Verification items for the finished model (mm, model axes). A direction names the side the tool comes from. Coordinates: 2 decimals unless noted, no trailing zeros. Loops run counter-clockwise (first coordinate to the right, second up) from the corner with the lowest first, then second, coordinate; pieces in that order, holes last. Notation, with made-up numbers: (-3, 71) - (5, 71) arc R15 ccw to (5, 78) - close; hole circle Ø7 at (78.25, -13). An arc over 180 degrees is marked (long way). Answer as CSV lines item,"result". Start each with the question number.
1. Gauge pin test, flat ends, axial feed: P1, Ø4, axis at x = 14.5, z = -12, coming from the +Y side; P2, Ø18.5, axis at x = 5.5, z = 4, coming from the -Y side. Record the tip position at first contact, or that the pin passes through.
2. Cross-section at A-A (x = 17). Enter the section's corners in (y, z), plus the area to 3 significant figures.
3. Cross-section at D-D (y = 10.5). Enter the section's corners in (x, z).
4. Set-up check for faces 4 (the flat face through (0, 3, -12.945)), 5 (the flat face through (23, 16, 16)), 6 (the flat face through (-26.25, 3, 0)), 7 (the cylindrical face through (-23.737, -4.93, -17.276)), 8 (the cylindrical face through (23.79, 10.93, 16.44)): record each of +Z, -Z, +X, -X, +Y, -Y from which the full face is reachable in a straight line by a thin tool's end or side.
5. Release check for a two-part mould opening along Z. For faces 1 (the flat face through (-23, -10, 8)), 2 (the flat face through (0, 3, 18.6)), 3 (the flat face through (21.25, 3, 0)) record: pulls with the +Z half, pulls with the -Z half, needs draft (parallel to the pull), parting line crosses it, or undercut.
6. Material ranges on line 1 (X direction, y = 4.75, z = 0); line 2 (Z direction, x = -12, y = 0.25); line 3 (Y direction, x = -20, z = 13.5), recorded low to high. Write a range as [from, to].
7. Cross-section at C-C (y = 2.5). Enter the section's corners in (x, z), plus the area to 3 significant figures.
8. Cross-section at B-B (z = -1). Enter the section's corners in (x, y).
Autodesk Inventor part; units mm, degrees
ref_plane "YZ Plane" through (0, 0, 0) normal (1, 0, 0) x (0, 1, 0)
ref_plane "XZ Plane" through (0, 0, 0) normal (0, 1, 0) x (-1, 0, 0)
ref_plane "XY Plane" through (0, 0, 0) normal (0, 0, 1) x (1, 0, 0)
sketch "Sketch1" plane through (0, 0, 0) normal (0, 1, 0) x (-1, 0, 0)
  line L0 (26.25, 18.6) -> (-26.25, 18.6)
  line L1 (-26.25, 18.6) -> (-26.25, -18.6)
  line L2 (-26.25, -18.6) -> (26.25, -18.6)
  line L3 (26.25, -18.6) -> (26.25, 18.6)
  line L4 (26.25, 18.6) -> (-26.25, -18.6) construction
  line L5 (-26.25, 18.6) -> (26.25, -18.6) construction
  line L6 (-26.25, -18.6) -> (-23.25, -18.6)
  point P0 (0, 0)
  dimension "d0" = 52.5
  dimension "d1" = 37.2
  dimension "d2" = 3
extrude "Extrusion1" add sketch "Sketch1" along normal blind 6
sketch "Sketch2" plane through (0, 6, 0) normal (0, 1, 0) x (1, 0, 0)
  line L0 (26.25, 18.6) -> (-26.25, 18.6)
  line L1 (26.25, 18.6) -> (26.25, 15.6)
  line L2 (26.25, -18.6) -> (26.25, 18.6)
  line L3 (26.25, 18.6) -> (23.25, 18.6)
  line L4 (23.25, 18.6) -> (23.25, 15.6)
  circle A0 centre (23.25, 15.6) radius 1
  line L5 (26.25, 0) -> (18.0402, 0)
  line L6 (0, 18.6) -> (0, 10.2391)
  circle A1 centre (23.25, -15.6) radius 1
  circle A2 centre (-23.25, 15.6) radius 1
  point P0 (0, 0)
  dimension "d5" = 3
  dimension "d6" = 3
  dimension "d7" = 2
extrude "Extrusion2" add sketch "Sketch2" along normal blind 10
sketch "Sketch4" plane through (0, 0, 0) normal (0, -1, 0) x (1, 0, 0)
  line L0 (26.25, -18.6) -> (-26.25, -18.6)
  line L1 (-26.25, -18.6) -> (-26.25, -16.6)
  line L2 (-26.25, -18.6) -> (-26.25, 18.6)
  line L3 (-26.25, -16.6) -> (-23, -16.6)
  circle A0 centre (-23, -16.6) radius 1
  line L4 (-23, -16.6) -> (-23, 8.4)
  line L5 (-23, -4.1) -> (-16.8136, -4.1)
  circle A1 centre (-23, 8.4) radius 1
  line L6 (0, -18.6) -> (0, -14.1147)
  circle A2 centre (23, -16.6) radius 1
  circle A3 centre (23, 8.4) radius 1
  point P0 (0, 0)
  dimension "d16" = 2
  dimension "d17" = 3.25
  dimension "d18" = 2
  dimension "d19" = 25
extrude "Extrusion4" add sketch "Sketch4" along normal blind 10
sketch "Sketch5" plane through (0, 6, 0) normal (0, 1, 0) x (1, 0, 0)
  line L0 (-21.2504, -12.9448) -> (21.2504, -12.9448)
  line L1 (21.2504, -12.9448) -> (21.2504, 12.9448)
  line L2 (21.2504, 12.9448) -> (-21.2504, 12.9448)
  line L3 (-21.2504, 12.9448) -> (-21.2504, -12.9448)
  line L4 (-21.2504, -12.9448) -> (21.2504, 12.9448) construction
  line L5 (21.2504, -12.9448) -> (-21.2504, 12.9448) construction
  point P0 (0, 0)
extrude "Extrusion5" cut sketch "Sketch5" against normal blind 10.5
properties part number "Divider_NodeMCU_Sipeed"
Values follow:
1,P1,"stops at y = 6"
1,P2,"stops at y = 0"
2,outline,"(0, -18.6) - (6, -18.6) - (6, -12.94) - (0, -12.94) - close; (0, 12.94) - (6, 12.94) - (6, 18.6) - (0, 18.6) - close"
2,area,"67.9 mm²"
3,outline,"circle Ø2 at (-23.25, -15.6); circle Ø2 at (23.25, -15.6); circle Ø2 at (23.25, 15.6)"
4,face 4,"+Y, -Y"
4,face 5,"+Z, -Z, +X, -X, +Y"
4,face 6,"+Z, -Z, -X, +Y, -Y"
4,face 7,"-Y"
4,face 8,"+Y"
5,face 1,"needs draft"
5,face 2,"pulls with the +Z half"
5,face 3,"undercut"
6,line 1,"x = [-26.25, -21.25], [21.25, 26.25]"
6,line 2,"z = [-18.6, -12.94], [12.94, 18.6]"
6,line 3,"y = [0, 6]"
7,outline,"(-26.25, -18.6) - (26.25, -18.6) - (26.25, 18.6) - (-26.25, 18.6) - close; hole (-21.25, -12.94) - (21.25, -12.94) - (21.25, 12.94) - (-21.25, 12.94) - close"
7,area,"853 mm²"
8,outline,"(-26.25, 0) - (-21.25, 0) - (-21.25, 6) - (-26.25, 6) - close; (21.25, 0) - (26.25, 0) - (26.25, 6) - (21.25, 6) - close"
